```python
from build123d import *

# Parameters (mm, degrees)
RESSALTO_EXTRUS_O1_DEPTH = 14.98
ESBO_O2_R                = 2
CORTE_EXTRUS_O1_DEPTH    = 62.5


with BuildPart() as part:
    # Esboço1 → Ressalto-extrusão1 (new body)
    with BuildSketch(Plane.XY):
        with BuildLine():
            Line((-17.493550541, 31.212986182), (-17.493550541, -98.787013818))
            Line((-17.493550541, -98.787013818), (19.286449459, -98.787013818))
            Line((19.286449459, -98.787013818), (19.286449459, 31.212986182))
            ThreePointArc((19.286449459, 31.212986182), (0.896449459, 49.602986182), (-17.493550541, 31.212986182))
        make_face()
    extrude(amount=RESSALTO_EXTRUS_O1_DEPTH)

    # Esboço2 → Corte-extrusão1 (cut, symmetric)
    with BuildSketch(Plane.XY.offset(14.98)):
        with Locations(Location((0, 36.56215444, 0), (0, 0, 180))):
            Circle(ESBO_O2_R)
    extrude(amount=CORTE_EXTRUS_O1_DEPTH, both=True, mode=Mode.SUBTRACT)


solid = part.part
```
Here's how the part is built. I have some questions about the finished solid (model axes, mm). Give positions to 0.01 mm unless a question says otherwise; leave off trailing zeros. Write each loop counter-clockwise with the first axis right and the second up, starting at its lowest first coordinate (ties: lowest second). Pieces come first, ordered by that corner, then holes. Notation, with made-up numbers: (49.25, 81) -> (85.25, 81) arc R31 ccw to (85.25, 114) -> close; hole circle Ø10 at (-18.75, 49.25). An arc over 180 degrees is marked (long way). Write each question's results on one line, items separated by ' | '.
Item 1: Suppose I cut it at C-C on x = -11. Write out the boundary of the cut face in (y, z), plus the area to 3 significant figures.
Output:
outline: (-98.79, 0) -> (45.24, 0) -> (45.24, 14.98) -> (-98.79, 14.98) -> close | area: 2,160 mm^2
Item 2: We'd pull the mould along Y, two halves only. Please class faces 1 (the face through (-0.92, 38.34, 7.59)), 2 (the face through (1, -98.787, 7)), 3 (the face through (1.3, 49.6, 7.4)), 4 (the face through (19.286, -35, 7)): pulls with the +Y half, pulls with the -Y half, needs draft (parallel to the pull), parting line crosses it, or undercut.
Output:
face 1: undercut | face 2: pulls with the -Y half | face 3: pulls with the +Y half | face 4: needs draft
Item 3: Suppose I cut it at A-A on x = 0. Write out the boundary of the cut face in (y, z), plus the area to 3 significant figures.
Output:
outline: (-98.79, 0) -> (34.56, 0) -> (34.56, 14.98) -> (-98.79, 14.98) -> close; (38.56, 0) -> (49.58, 0) -> (49.58, 14.98) -> (38.56, 14.98) -> close | area: 2,160 mm^2
Item 4: If I drill on L1, parallel to Y at x = 0, z = 7.25; L2, parallel to Y at x = -12, z = 13; L3, parallel to Y at x = 1.5, z = 8.75, over which ranges is the centre line in solid material (lowest first)?
Output:
L1: y = -98.79 to 34.56, 38.56 to 49.58 | L2: y = -98.79 to 44.32 | L3: y = -98.79 to 35.24, 37.89 to 49.59
Item 5: For pin 1 Ø2.5 at (x, y) = (0, 36.56) entering from +Z; pin 2 Ø3 at (x, z) = (13.5, 1.5) entering from +Y, each with a flat end and sliding along its axis, tell me the tip position at first contact or that it passes through.
Output:
pin 1: passes through | pin 2: stops at y = 45.87
Item 6: Suppose I cut it at B-B on z = 6.25. Write out the boundary of the cut face in (x, y), plus the area to 3 significant figures.
Output:
outline: (-17.49, -98.79) -> (19.29, -98.79) -> (19.29, 31.21) arc R18.39 ccw to (-17.49, 31.21) -> close; hole circle Ø4 at (0, 36.56) | area: 5,300 mm^2
